Autodesk Inventor part; units mm, degrees
ref_plane "YZ Plane" through (0, 0, 0) normal (1, 0, 0) x (0, 1, 0)
ref_plane "XZ Plane" through (0, 0, 0) normal (0, 1, 0) x (-1, 0, 0)
sketch "Sketch1" plane through (0, 0, 0) normal (0, 1, 0) x (-1, 0, 0)
  line L0 (152.4, 12.7) -> (-152.4, 12.7)
  line L1 (-152.4, 12.7) -> (-152.4, -12.7)
  line L2 (-152.4, -12.7) -> (152.4, -12.7)
  line L3 (152.4, -12.7) -> (152.4, 12.7)
  line L4 (152.4, 12.7) -> (-152.4, -12.7) construction
  line L5 (-152.4, 12.7) -> (152.4, -12.7) construction
  point P0 (0, 0)
  dimension "d0" = 304.8
  dimension "d1" = 25.4
extrude "Extrusion1" add sketch "Sketch1" along normal mid plane 25.4
sketch "Sketch3" plane through (0, 12.7, 0) normal (0, 1, 0) x (1, 0, 0)
  line L0 (-152.4, -6.858) -> (88.9, -6.858)
  line L1 (88.9, -6.858) -> (88.9, 6.858)
  line L2 (88.9, 6.858) -> (-152.4, 6.858)
  line L3 (-152.4, 6.858) -> (-152.4, -6.858)
  line L4 (-152.4, -6.858) -> (88.9, 6.858) construction
  line L5 (88.9, -6.858) -> (-152.4, 6.858) construction
  line L6 (-152.4, 12.7) -> (-152.4, -12.7)
  point P0 (0, 0)
  point P1 (-31.75, 0)
  dimension "d7" = 0
  dimension "d8" = 13.716
  dimension "d9" = 241.3
extrude "Extrusion2" cut sketch "Sketch3" against normal through all
sketch "Sketch4" plane through (0, 12.7, 0) normal (0, 1, 0) x (1, 0, 0)
  line L0 (152.4, 12.7) -> (-152.4, 12.7)
  line L1 (152.4, 12.7) -> (114.3, 12.7)
  line L2 (114.3, 12.7) -> (114.3, 6.35)
  line L3 (114.3, 6.35) -> (152.4, 6.35)
  line L4 (152.4, 6.35) -> (152.4, 12.7)
  line L5 (152.4, 0) -> (88.9, 0) construction
  line L6 (88.9, 6.858) -> (88.9, -6.858) construction
  point P0 (0, 0)
  point P1 (114.3, 12.7)
  dimension "d12" = 38.1
  dimension "d13" = 6.35
extrude "Extrusion3" cut sketch "Sketch4" against normal through all
mirror "Mirror1" about plane through (0, 0, 0) normal (0, 0, 1) of "Extrusion3"
sketch "Sketch5" plane through (-152.4, -12.7, 12.7) normal (0, 0, 1) x (1, 0, 0)
  circle A0 centre (12.7, 12.7) radius 5.2705
  circle A1 centre (292.1, 12.7) radius 5.2705
  line L0 (0, 25.4) -> (0, 0)
  line L1 (304.8, 25.4) -> (304.8, 0)
  point P0 (152.4, 12.7)
  dimension "d16" = 10.541
  dimension "d17" = 12.7
  dimension "d18" = 12.7
extrude "Extrusion4" cut sketch "Sketch5" against normal through all
properties part number "connectingRodV03-8-in" material "PET Plastic"
Input: part model. Units: mm. Frame: model coordinates. A direction names the side the tool comes from. Give positions to 0.01 mm unless a question says otherwise; leave off trailing zeros. Loops run counter-clockwise (first coordinate to the right, second up) from the corner with the lowest first, then second, coordinate; pieces in that order, holes last.
1) Section query A-A on y = 0. Return the cut outline in (x, z).
A:
outline: (-152.4, -12.7) - (-144.97, -12.7) - (-144.97, -6.86) - (-152.4, -6.86) - close; (-152.4, 6.86) - (-144.97, 6.86) - (-144.97, 12.7) - (-152.4, 12.7) - close; (-134.43, -12.7) - (114.3, -12.7) - (114.3, -6.35) - (134.43, -6.35) - (134.43, 6.35) - (114.3, 6.35) - (114.3, 12.7) - (-134.43, 12.7) - (-134.43, 6.86) - (88.9, 6.86) - (88.9, -6.86) - (-134.43, -6.86) - close; (144.97, -6.35) - (152.4, -6.35) - (152.4, 6.35) - (144.97, 6.35) - close
2) Section query B-B on x = -11.5. Return the cut outline in (y, z), and give its area (3 significant figures).
A:
outline: (-12.7, -12.7) - (12.7, -12.7) - (12.7, -6.86) - (-12.7, -6.86) - close; (-12.7, 6.86) - (12.7, 6.86) - (12.7, 12.7) - (-12.7, 12.7) - close
area: 297 mm2
3) Contact query for flat-ended pins moving along their axis: pin 1 (9.5 mm diameter, centred on x = 139.7, y = 0, fed in from -Z); pin 2 (15 mm diameter, centred on y = 6, z = 3, fed in from -X); pin 3 (7 mm diameter, centred on y = 2, z = 10, fed in from +X); pin 4 (8 mm diameter, centred on y = 6, z = -1, fed in from -X). Output: stop coordinate, or through.
A:
pin 1: passes through
pin 2: stops at x = -152.4
pin 3: stops at x = 114.3
pin 4: stops at x = 88.9
4) Section query D-D on x = 139.7. Return the cut outline in (y, z), and give its area (3 significant figures).
A:
outline: (-12.7, -6.35) - (-5.27, -6.35) - (-5.27, 6.35) - (-12.7, 6.35) - close; (5.27, -6.35) - (12.7, -6.35) - (12.7, 6.35) - (5.27, 6.35) - close
area: 189 mm2
5) Mould query, pull axis X, two halves, no side actions, for faces 1 (the flat face through (134, 0, 6.35)), 2 (the cylindrical face through (-143.88, -3.21, -9.74)), 3 (the flat face through (152.4, 0, 0)). Classes: released by +X, released by -X, zero draft, split by the parting line, or undercut.
A:
face 1: zero draft
face 2: undercut
face 3: released by +X
6) Reachability of faces 4 (the flat face through (-152.4, 0, 10)), 5 (the flat face through (-30, 0, -6.858)), 6 (the flat face through (114.3, 0, 9)), 7 (the flat face through (133, 0, -6.35)) from +Z, -Z, +X, -X, +Y, -Y: full face, straight path, thin tool, end or side. Return the list, or none.
A:
face 4: +Z, -Z, -X, +Y, -Y
face 5: -X, +Y, -Y
face 6: +Z, +X, +Y, -Y
face 7: -Z, +X, +Y, -Y
7) Line query: L1, parallel to Z at x = 10.5, y = -8; L2, parallel to Y at x = -139.7, z = -9.6; L3, parallel to Z at x = 124, y = -3.5. Output: solid intervals per line, ascending.
A:
L1: z = -12.7 to -6.86, 6.86 to 12.7
L2: y = -12.7 to -5.27, 5.27 to 12.7
L3: z = -6.35 to 6.35
8) Section query C-C on x = -139.7. Return the cut outline in (y, z), and give its area (3 significant figures).
A:
outline: (-12.7, -12.7) - (-5.27, -12.7) - (-5.27, -6.86) - (-12.7, -6.86) - close; (-12.7, 6.86) - (-5.27, 6.86) - (-5.27, 12.7) - (-12.7, 12.7) - close; (5.27, -12.7) - (12.7, -12.7) - (12.7, -6.86) - (5.27, -6.86) - close; (5.27, 6.86) - (12.7, 6.86) - (12.7, 12.7) - (5.27, 12.7) - close
area: 174 mm2
